```python
from build123d import *

# Parameters (mm, degrees)
F0_R      = 6
F1_DEPTH  = 30
F2_R      = 2.75
F3_DEPTH  = 30.001
F8_R      = 5
F8_R_2    = 1.6
F9_DEPTH  = 2
F12_W     = 4
F12_H     = 30
F13_DEPTH = 3
F14_R     = 2.5
F15_DEPTH = 3.5


with BuildPart() as f1:
    # F0 (on Front) → F1 (new body)
    with BuildSketch(Plane.XZ):
        Circle(F0_R)
    extrude(amount=F1_DEPTH)

    # F2 (on face) → F3 (cut, through all)
    with BuildSketch(Plane.XZ.offset(30)):
        Circle(F2_R)
    extrude(amount=-F3_DEPTH, mode=Mode.SUBTRACT)

    # F8 (on face) → F9 (join)
    with BuildSketch(Plane.XZ.offset(30)):
        Circle(F8_R)
        Circle(F8_R_2, mode=Mode.SUBTRACT)
    extrude(amount=-F9_DEPTH)

    # F12 (on offset) → F13 (cut)
    with BuildSketch(Plane.XY.offset(4)):
        with Locations((0, -15)):
            Rectangle(F12_W, F12_H)
    extrude(amount=F13_DEPTH, mode=Mode.SUBTRACT)

    # F14 (on offset) → F15 (cut)
    with BuildSketch(Plane.YZ.offset(6)):
        with Locations((-25, 0)):
            Circle(F14_R)
    extrude(amount=-F15_DEPTH, mode=Mode.SUBTRACT)


solid = f1.part
```
CAD build for the part. Positions are in the model's coordinates, mm. A direction names the side the tool comes from. Round coordinates to 2 decimals unless told otherwise and drop trailing zeros. Order: outer loops, then holes, each group sorted by start corner. A loop starts at its lowest first (then second) coordinate and runs counter-clockwise, first axis right, second up. Notation, with made-up numbers: (13.25, 37) - (70.25, 37) arc R12 ccw to (70.25, 49) - close; hole circle Ø9 at (81, -7). An arc over 180 degrees is marked (long way). Answer in a Markdown table with one row per item. Add a question column.
(1) Band-saw the part on B-B on z = 0. List the corners of the cut face in (x, y), and give its area (3 significant figures).
(2) Band-saw the part on A-A on x = 0. List the corners of the cut face in (y, z), and give its area (3 significant figures).
(3) Band-saw the part on C-C on y = -6.5. List the corners of the cut face in (x, z), and give its area (3 significant figures).
(4) Drop flat-ended pins along their axis: pin 1 Ø2 at (x, y) = (-3, -25.5) entering from -Z; pin 2 Ø3 at (x, y) = (1.5, -4) entering from +Z; pin 3 Ø0.5 at (y, z) = (-11.5, 4.5) entering from -X; pin 4 Ø4.5 at (x, z) = (-0.5, -0.5) entering from +Y. Give the stop position or say it passes through.
(5) 3-axis set-ups, long thin cutter, end or side, ignore diameter. For faces 1 (the face through (2.5, -25, 2)), 2 (the face through (-1.27, -29.01, -0.97)), 3 (the face through (-2.747, -14.196, 0.121)), 4 (the face through (0, -15, 4)): which of +Z, -Z, +X, -X, +Y, -Y reach the whole face in a straight line?
(6) Band-saw the part on D-D on y = -25. List the corners of the cut face in (x, z), and give its area (3 significant figures).
(7) Mould opens along X. For faces 5 (the face through (-2, -15, 5)), 6 (the face through (0, -15, -6)), 7 (the face through (4.27, -22.69, -0.96)) say: +X half, -X half, draft (parallel to the pull), parting line (faces both ways), or undercut.
(8) Probe L1, parallel to Z at x = 0, y = -28.6; L2, parallel to Y at x = 5.2, z = 0; L3, parallel to Z at x = 0, y = -13.5. List the from-to ranges inside material, lowest first. Write a range as [from, to].
Data:
| question | item | result |
|---|---|---|
| 1 | outline | (-6, -30) - (-1.6, -30) - (-1.6, -28) - (-2.75, -28) - (-2.75, 0) - (-6, 0) - close; (1.6, -30) - (6, -30) - (6, -27.5) - (2.75, -27.5) - (2.75, -28) - (1.6, -28) - close; (2.75, -22.5) - (6, -22.5) - (6, 0) - (2.75, 0) - close |
| 1 | area | 183 mm^2 |
| 2 | outline | (-30, -6) - (0, -6) - (0, -2.75) - (-28, -2.75) - (-28, -1.6) - (-30, -1.6) - close; (-30, 1.6) - (-28, 1.6) - (-28, 2.75) - (0, 2.75) - (0, 4) - (-30, 4) - close |
| 2 | area | 140 mm^2 |
| 3 | outline | (-2, 4) - (-2, 5.66) arc R6 ccw (long way) to (2, 5.66) - (2, 4) - close; hole circle Ø5.5 at (0, 0) |
| 3 | area | 81.8 mm^2 |
| 4 | pin 1 | stops at z = -5.66 |
| 4 | pin 2 | stops at z = 5.66 |
| 4 | pin 3 | stops at x = -4.24 |
| 4 | pin 4 | stops at y = 0 |
| 5 | face 1 | +X |
| 5 | face 2 | +Y, -Y |
| 5 | face 3 | +Y |
| 5 | face 4 | +Z, +Y, -Y |
| 6 | outline | (-2, 4) - (-2, 5.66) arc R6 ccw (long way) to (5.45, -2.5) - (2.5, -2.5) - (2.5, -1.15) arc R2.75 cw (long way) to (2.5, 1.15) - (2.5, 2.5) - (5.45, 2.5) arc R6 ccw to (2, 5.66) - (2, 4) - close |
| 6 | area | 65.6 mm^2 |
| 7 | face 5 | undercut |
| 7 | face 6 | parting line |
| 7 | face 7 | draft |
| 8 | L1 | z = [-6, -1.6], [1.6, 4] |
| 8 | L2 | y = [-30, -27.5], [-22.5, 0] |
| 8 | L3 | z = [-6, -2.75], [2.75, 4] |
